Geometry check sheet. Reference: the model listing, model coordinates, mm. Coordinates: 2 decimals unless noted, no trailing zeros. Write each loop counter-clockwise with the first axis right and the second up, starting at its lowest first coordinate (ties: lowest second). Pieces come first, ordered by that corner, then holes.
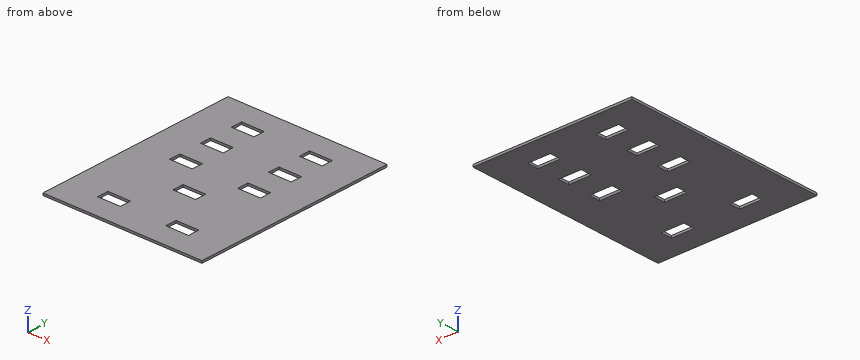
from build123d import *

# Parameters (mm, degrees)
SKETCH1_W           = 350
SKETCH1_H           = 450
BOSS_EXTRUDE1_DEPTH = 5
SKETCH2_W           = 50
SKETCH2_H           = 25
CUT_EXTRUDE1_DEPTH  = 571.109638578


with BuildPart() as part:
    # Sketch1 → Boss-Extrude1 (new body)
    with BuildSketch(Plane.XY):
        with Locations((175, 225)):
            Rectangle(SKETCH1_W, SKETCH1_H)
    extrude(amount=BOSS_EXTRUDE1_DEPTH)

    # Sketch2 → Cut-Extrude1 (cut, through all)
    with BuildSketch(Plane.XY.offset(5)):
        with Locations((100, 387.5)):
            Rectangle(SKETCH2_W, SKETCH2_H)
    cut_extrude1 = extrude(amount=-CUT_EXTRUDE1_DEPTH, mode=Mode.SUBTRACT)

    # Sketch-Pattern1: Cut-Extrude1 at 8 more places
    with Locations((150, 0, 0), (150, -75, 0), (0, -75, 0), (0, -150, 0), (150, -150, 0), (75, -225, 0), (0, -325, 0), (150, -325, 0)):
        add(cut_extrude1, mode=Mode.SUBTRACT)


solid = part.part
1. Gauge pin test, flat end, axial feed: pin 1 Ø2.5 at (x, z) = (240, 2) entering from -Y. Record the tip position at first contact, or that the pin passes through.
Computed values:
pin 1: stops at y = 0
2. Sectioned sample at B-B, the plane y = 319. Record the boundary of the cut face in (x, z).
Computed values:
outline: (0, 0) - (75, 0) - (75, 5) - (0, 5) - close; (125, 0) - (225, 0) - (225, 5) - (125, 5) - close; (275, 0) - (350, 0) - (350, 5) - (275, 5) - close
3. Thickness scan on line 1 along Y through (x, z) = (259.5, 2.55); line 2 along X through (y, z) = (249, 4.05); line 3 along Y through (x, z) = (199, 4.75). Record the ranges inside material, lowest first.
Computed values:
line 1: y = 0 to 50, 75 to 225, 250 to 300, 325 to 375, 400 to 450
line 2: x = 0 to 75, 125 to 225, 275 to 350
line 3: y = 0 to 150, 175 to 450
4. Sectioned sample at C-C, the plane z = 1.35. Give the number of separate pieces and of enclosed holes in the cut face, and give its area (3 significant figures).
Computed values:
separate pieces: 1
enclosed holes: 9
area: 146,000 mm2
5. Sectioned sample at A-A, the plane x = 80. Record the boundary of the cut face in (y, z), and give its area (3 significant figures).
Computed values:
outline: (0, 0) - (50, 0) - (50, 5) - (0, 5) - close; (75, 0) - (225, 0) - (225, 5) - (75, 5) - close; (250, 0) - (300, 0) - (300, 5) - (250, 5) - close; (325, 0) - (375, 0) - (375, 5) - (325, 5) - close; (400, 0) - (450, 0) - (450, 5) - (400, 5) - close
area: 1,750 mm2
